```python
from build123d import *

# Parameters (mm, degrees)
F1_DEPTH = 175


with BuildPart() as f1:
    # F0 (on Right) → F1 (new body, symmetric)
    with BuildSketch(Plane.YZ):
        with BuildLine():
            ThreePointArc((42.5, 5), (41.035534, 8.535534), (37.5, 10))
            Line((37.5, 10), (-37.5, 10))
            ThreePointArc((-37.5, 10), (-41.035534, 8.535534), (-42.5, 5))
            Line((-42.5, 5), (-42.5, -5))
            ThreePointArc((-42.5, -5), (-41.035534, -8.535534), (-37.5, -10))
            Line((-37.5, -10), (37.5, -10))
            ThreePointArc((37.5, -10), (41.035534, -8.535534), (42.5, -5))
            Line((42.5, -5), (42.5, 5))
        make_face()
    extrude(amount=F1_DEPTH, both=True)


solid = f1.part
```
Work out the finished part from the listing and answer in its coordinate system (mm). Give positions to 0.01 mm unless a question says otherwise; leave off trailing zeros. One line per question, with ' | ' between items.
(1) The mould has two halves that part along X. Classify faces 1 (the face through (-175, -1, 0)), 2 (the face through (2, 1, 10)), 3 (the face through (175, -1, 0)): +X half, -X half, draft (parallel to the pull), parting line (faces both ways), or undercut.
Recorded:
face 1: -X half | face 2: draft | face 3: +X half
(2) Straight lines are drawn through the part: probe 1 along Z at (x, y) = (-123.5, -38); probe 2 along Y at (x, z) = (67.5, 7); probe 3 along Y at (x, z) = (-117.5, -6). For each, find the intervals that lie inside material, in ascending order.
Recorded:
probe 1: z = -9.97 to 9.97 | probe 2: y = -42.08 to 42.08 | probe 3: y = -42.4 to 42.4
(3) This flat-tipped pin is pushed along its axis until it touches: pin 1 Ø1.5 at (x, z) = (-71, 6.5) entering from -Y. Where does it stop, or does it pass through?
Recorded:
pin 1: stops at y = -42.44
